```python
from build123d import *

# Parameters (mm, degrees)
SKETCH2_W                   = 110.49
SKETCH2_H                   = 6.35
BOSS_EXTRUDE1_DEPTH         = 63.5
SKETCH3_R                   = 14.2875
CUT_EXTRUDE1_DEPTH          = 85.407242136
CHAMFER1_SIZE               = 6.35
CUT_EXTRUDE2_DEPTH          = 1.524
TAP_DRILL_FOR_M4X0_7_TAP1_D = 3.3
TAP_DRILL_FOR_M7X1_0_TAP1_D = 6
FILLET2_R                   = 0.762


with BuildPart() as part:
    # Sketch2 → Boss-Extrude1 (new body)
    with BuildSketch(Plane(origin=(0, 0, 0), x_dir=(1, 0, 0), z_dir=(0, 1, 0))):
        Rectangle(SKETCH2_W, SKETCH2_H)
    extrude(amount=-BOSS_EXTRUDE1_DEPTH)

    # Sketch3 → Cut-Extrude1 (cut, through all)
    with BuildSketch(Plane.XY.offset(3.175)):
        with Locations((0, -28.8150046)):
            Circle(SKETCH3_R)
    extrude(amount=-CUT_EXTRUDE1_DEPTH, mode=Mode.SUBTRACT)

    # Chamfer1
    chamfer1_edges = [part.edges().sort_by_distance(p)[0] for p in [
        (55.245, 0, 0),
        (-55.245, 0, 0),
    ]]
    chamfer(chamfer1_edges, length=CHAMFER1_SIZE)

    # Sketch12 → Cut-Extrude2 (cut)
    with BuildSketch(Plane.XY.offset(3.175)):
        with BuildLine():
            Line((-33.655, -49.5), (-33.655, -63.5))
            Line((-33.655, -63.5), (-18.655, -63.5))
            Line((-18.655, -63.5), (-18.655, -49.5))
            ThreePointArc((-18.655, -49.5), (-26.155, -42), (-33.655, -49.5))
        make_face()
    cut_extrude2 = extrude(amount=-CUT_EXTRUDE2_DEPTH, mode=Mode.SUBTRACT)

    # Mirror1: Cut-Extrude2 across plane
    add(cut_extrude2.mirror(Plane(origin=(0, 0, 0), x_dir=(0, 0, 1), z_dir=(1, 0, 0))), mode=Mode.SUBTRACT)

    # Tap Drill for M4x0.7 Tap1 (through all)
    with Locations(Plane.XY.offset(3.175)):
        with Locations((-26.155, -50), (26.155, -50)):
            Hole(TAP_DRILL_FOR_M4X0_7_TAP1_D / 2)

    # Tap Drill for M7x1.0 Tap1 (through all)
    with Locations(Plane(origin=(0, 0, -3.175), x_dir=(-1, 0, 0), z_dir=(0, 0, -1))):
        with Locations((44.245, -26), (44.245, -51), (-44.245, -51), (-44.245, -26)):
            Hole(TAP_DRILL_FOR_M7X1_0_TAP1_D / 2)

    # Fillet2
    fillet2_edges = [part.edges().sort_by_distance(p)[0] for p in [
        (55.245, -63.5, 0),
        (0, -63.5, -3.175),
        (0, 0, 3.175),
        (0, 0, -3.175),
        (48.895, 0, 0),
        (-48.895, 0, 0),
        (52.07, -3.175, 3.175),
        (-52.07, -3.175, 3.175),
        (-55.245, -6.35, 0),
        (52.07, -3.175, -3.175),
        (-52.07, -3.175, -3.175),
        (55.245, -6.35, 0),
        (0, -63.5, 3.175),
        (-26.155, -63.5, 1.651),
        (-18.655, -63.5, 2.413),
        (-33.655, -63.5, 2.413),
        (44.45, -63.5, 3.175),
        (-55.245, -63.5, 0),
        (33.655, -63.5, 2.413),
        (18.655, -63.5, 2.413),
        (26.155, -63.5, 1.651),
        (-55.245, -34.925, -3.175),
        (55.245, -34.925, -3.175),
        (55.245, -34.925, 3.175),
        (-55.245, -34.925, 3.175),
        (-44.45, -63.5, 3.175),
    ]]
    fillet(fillet2_edges, radius=FILLET2_R)


solid = part.part
```
Design review of the part built by this model. Coordinates are the model's own, in mm. A direction names the side the tool comes from. Give positions to 0.01 mm unless a question says otherwise; leave off trailing zeros. Loops run counter-clockwise (first coordinate to the right, second up) from the corner with the lowest first, then second, coordinate; pieces in that order, holes last. Notation, with made-up numbers: M 8.25,66.5 L 49.25,66.5 A19 ccw 49.25,85.5 Z; hole C -6.5,78 d2. An arc over 180 degrees is marked long. Return JSON: item names as keys, results as strings. Group by question number.
Item 1: We need section C-C (y = -26). Give the boundary of the cut face in (x, z) (3 decimals), and give its area (3 significant figures).
Item 2: We need section B-B (y = -38). Give the boundary of the cut face in (x, z) (3 decimals).
Item 3: Insertion check: pin 1 Ø1.7 at (y, z) = (-57, 2.5) entering from -X (3 decimals); pin 2 Ø5 at (x, y) = (44.245, -51) entering from +Z; pin 3 Ø12 at (x, y) = (25.5, -57.5) entering from +Z. Each pin has a flat end and moves straight along its axis. Give the tip position at first contact, or say it passes through.
Item 4: Tool access review of faces 1 (the flat face through (26, -52, 1.651)), 2 (the flat face through (55.245, -34, 0)): name each direction out of +Z, -Z, +X, -X, +Y, -Y from which nothing blocks a thin tool from reaching the whole face with its end or side.
Item 5: For probe 1 along Y at (x, z) = (0, 0.75); probe 2 along Y at (x, z) = (-10, 3); probe 3 along X at (y, z) = (-33, -2) (3 decimals), list the stretches that pass through material, from the lowest coordinate up.
Item 6: Mouldability with a two-part tool opening along Y and no side actions: class faces 3 (the flat face through (-26, -52, 1.651)), 4 (the cylindrical face through (51.95, -3.38, -2.96)), 5 (the cylindrical face through (-44.636, -48.026, 0.044)) as released by +Y, released by -Y, zero draft, split by the parting line, or undercut.
Item 7: We need section A-A (x = 26.5). Give the boundary of the cut face in (y, z) (3 decimals), and give its area (3 significant figures).
Item 8: We need section D-D (y = -19.5). Give the boundary of the cut face in (x, z) (3 decimals), and give its area (3 significant figures).
Output:
{
 "1": {"outline": "M -55.245,-2.413 A0.762 ccw -54.483,-3.175 L -47.245,-3.175 L -47.245,3.175 L -54.483,3.175 A0.762 ccw -55.245,2.413 Z; M -41.245,-3.175 L -14.007,-3.175 L -14.007,3.175 L -41.245,3.175 Z; M 14.007,-3.175 L 41.245,-3.175 L 41.245,3.175 L 14.007,3.175 Z; M 47.245,-3.175 L 54.483,-3.175 A0.762 ccw 55.245,-2.413 L 55.245,2.413 A0.762 ccw 54.483,3.175 L 47.245,3.175 Z", "area": "447 mm^2"},
 "2": {"outline": "M -55.245,-2.413 A0.762 ccw -54.483,-3.175 L -10.944,-3.175 L -10.944,3.175 L -54.483,3.175 A0.762 ccw -55.245,2.413 Z; M 10.944,-3.175 L 54.483,-3.175 A0.762 ccw 55.245,-2.413 L 55.245,2.413 A0.762 ccw 54.483,3.175 L 10.944,3.175 Z"},
 "3": {"pin 1": "stops at x = -55.245", "pin 2": "passes through", "pin 3": "stops at z = 1.65"},
 "4": {"face 1": "+Z, -Y", "face 2": "+Z, -Z, +X, +Y, -Y"},
 "5": {"probe 1": "y = -63.5 to -43.1, -14.53 to 0", "probe 2": "y = -63.22 to -39.02, -18.61 to -0.28", "probe 3": "x = -55.245 to -13.661, 13.661 to 55.245"},
 "6": {"face 3": "zero draft", "face 4": "released by +Y", "face 5": "undercut"},
 "7": {"outline": "M -63.5,-2.413 A0.762 ccw -62.738,-3.175 L -51.614,-3.175 L -51.614,1.651 L -62.738,1.651 A0.762 ccw -63.5,0.889 Z; M -48.386,-3.175 L -0.762,-3.175 A0.762 ccw 0,-2.413 L 0,2.413 A0.762 ccw -0.762,3.175 L -42.008,3.175 L -42.008,1.651 L -48.386,1.651 Z", "area": "354 mm^2"},
 "8": {"outline": "M -55.245,-2.413 A0.762 ccw -54.483,-3.175 L -10.833,-3.175 L -10.833,3.175 L -54.483,3.175 A0.762 ccw -55.245,2.413 Z; M 10.833,-3.175 L 54.483,-3.175 A0.762 ccw 55.245,-2.413 L 55.245,2.413 A0.762 ccw 54.483,3.175 L 10.833,3.175 Z", "area": "564 mm^2"}
}
